Check sheet for the modelled part. Datum: model origin and axes. Units: mm. A direction names the side the tool comes from. Round coordinates to 2 decimals unless told otherwise and drop trailing zeros. Write each loop counter-clockwise with the first axis right and the second up, starting at its lowest first coordinate (ties: lowest second). Pieces come first, ordered by that corner, then holes.
Item 1: Go/stop test with flat-tipped pins: pin 1 Ø1 at (x, z) = (0, 6) entering from +Y; pin 2 Ø5 at (x, z) = (-4.5, 2.5) entering from -Y. Record where each tip stops, or that it passes through.
Item 2: Material ranges on line 1 (Y direction, x = 0, z = 4); line 2 (Z direction, x = 7.25, y = -5.5); line 3 (Y direction, x = 6, z = 1.75), recorded low to high.
Item 3: Cross-section at D-D on z = 10.75. Enter the section's corners in (x, y), plus the area to 3 significant figures.
Item 4: Release check for a two-part mould opening along Y. For faces 1 (the flat face through (-1.42, -3.92, 12)), 2 (the cylindrical face through (-6, 0, 7)), 3 (the cylindrical face through (0.867, -3.905, 5.916)) record: +Y half, -Y half, draft (parallel to the pull), parting line (faces both ways), or undercut.
Item 5: Cross-section at A-A on y = 0. Enter the section's corners in (x, z).
Item 6: Tool access check on faces 4 (the flat face through (5, -5, 2)), 5 (the cylindrical face through (-4.42, -6.14, 0.99)). Record the directions out of +Z, -Z, +X, -X, +Y, -Y that give a thin tool (end or side, any length) a straight path to the whole face; none if there is none.
Item 7: Cross-section at C-C on y = 3.5. Enter the section's corners in (x, z).
from build123d import *

# Parameters (mm, degrees)
SKETCH1_R           = 11
SKETCH1_R_2         = 1.85
BOSS_EXTRUDE1_DEPTH = 2
SKETCH2_R           = 6
BOSS_EXTRUDE2_DEPTH = 10
SKETCH4_R           = 4
CUT_EXTRUDE1_DEPTH  = 15


with BuildPart() as part:
    # Sketch1 → Boss-Extrude1 (new body)
    with BuildSketch(Plane(origin=(0, 0, 0), x_dir=(0, 1, 0), z_dir=(0, 0, 1))):
        with Locations(Location((0, 0, 0), (0, 0, 270))):
            Circle(SKETCH1_R)
        with Locations(Location((-7.392247164, 3.058542441, 0), (0, 0, 270))):
            Circle(SKETCH1_R_2, mode=Mode.SUBTRACT)
        with Locations(Location((3.058542441, 7.392247164, 0), (0, 0, 270))):
            Circle(SKETCH1_R_2, mode=Mode.SUBTRACT)
        with Locations(Location((7.392247164, -3.058542441, 0), (0, 0, 270))):
            Circle(SKETCH1_R_2, mode=Mode.SUBTRACT)
        with Locations(Location((-3.058542441, -7.392247164, 0), (0, 0, 270))):
            Circle(SKETCH1_R_2, mode=Mode.SUBTRACT)
    extrude(amount=BOSS_EXTRUDE1_DEPTH)

    # Sketch2 → Boss-Extrude2 (add)
    with BuildSketch(Plane.XY.offset(2)):
        Circle(SKETCH2_R)
    extrude(amount=BOSS_EXTRUDE2_DEPTH)

    # Sketch4 → Cut-Extrude1 (cut)
    with BuildSketch(Plane(origin=(0, 0, 0), x_dir=(1, 0, 0), z_dir=(0, 0, -1))):
        with Locations(Location((0, 0, 0), (0, 0, 180))):
            Circle(SKETCH4_R)
    extrude(amount=-CUT_EXTRUDE1_DEPTH, mode=Mode.SUBTRACT)


solid = part.part
Response values:
1. pin 1: stops at y = 6
1. pin 2: stops at y = -10.81
2. line 1: y = -6 to -4, 4 to 6
2. line 2: z = 0 to 2
2. line 3: y = -9.22 to -4.28, -1.84 to 9.22
3. outline: circle Ø12 at (0, 0); hole circle Ø8 at (0, 0)
3. area: 62.8 mm2
4. face 1: draft
4. face 2: parting line
4. face 3: undercut
5. outline: (-11, 0) - (-4, 0) - (-4, 12) - (-6, 12) - (-6, 2) - (-11, 2) - close; (4, 0) - (11, 0) - (11, 2) - (6, 2) - (6, 12) - (4, 12) - close
6. face 4: +Z
6. face 5: +Z, -Z
7. outline: (-10.43, 0) - (-9.19, 0) - (-9.19, 2) - (-10.43, 2) - close; (-5.6, 0) - (-1.94, 0) - (-1.94, 12) - (-4.87, 12) - (-4.87, 2) - (-5.6, 2) - close; (1.94, 0) - (10.43, 0) - (10.43, 2) - (4.87, 2) - (4.87, 12) - (1.94, 12) - close
